CAD build for the part. Positions are in the model's coordinates, mm. A direction names the side the tool comes from. Give positions to 0.01 mm unless a question says otherwise; leave off trailing zeros. Write each loop counter-clockwise with the first axis right and the second up, starting at its lowest first coordinate (ties: lowest second). Pieces come first, ordered by that corner, then holes. Notation, with made-up numbers: (-17, 62.25) -> (39, 62.25) arc R12 cw to (39, 77.25) -> close; hole circle Ø7 at (8, 36.25). An arc over 180 degrees is marked (long way). Answer in a Markdown table with one row per item. Add a question column.
```python
from build123d import *

# Parameters (mm, degrees)
SKETCH_1_W   = 40
SKETCH_1_H   = 10
SKETCH_1_W_2 = 20
SKETCH_1_H_2 = 40
SKETCH_1_H_3 = 2.5


with BuildPart() as part:
    # 草圖1 → 旋轉1 (revolve)
    with BuildSketch(Plane.XY, mode=Mode.PRIVATE) as revolve_1_sk:
        with Locations((-20, 25)):
            Rectangle(SKETCH_1_W, SKETCH_1_H)
        with Locations((10, 20)):
            Rectangle(SKETCH_1_W_2, SKETCH_1_H_2)
        Polygon((20, 25), (20, 0), (40, 0), (40, 20), (40, 25), align=None)
        Polygon((40, 20), (40, 0), (60, 0), (60, 15), (60, 20), align=None)
        Polygon((60, 15), (60, 0), (80, 0), (80, 10), (80, 15), align=None)
        Polygon((80, 10), (80, 0), (100, 0), (100, 5), (100, 10), align=None)
        Polygon((100, 5), (100, 0), (120, 0), (120, 2.5), (120, 5), align=None)
        with Locations((130, 1.25)):
            Rectangle(SKETCH_1_W_2, SKETCH_1_H_3)
    revolve(revolve_1_sk.sketch.rotate(Axis((0, 0, 0), (1, 0, 0)), 90), axis=Axis((0, 0, 0), (1, 0, 0)))


solid = part.part
```
Item 1: Slice it at C-C, the plane x = 114.5. List the corners of the cut face in (y, z), then the cut area to 3 significant figures.
Item 2: Slice it at D-D, the plane y = 34. List the corners of the cut face in (x, z).
Item 3: Probe L1, parallel to Y at x = -16.5, z = 0; L2, parallel to Z at x = -3.5, y = -16; L3, parallel to X at y = -22.5, z = -28.5. List the from-to ranges inside material, lowest first. Write a range as from..to.
Item 4: Which spindle directions (+Z, -Z, +X, -X, +Y, -Y) get a long thin tool onto all of the face, cutting with end or side? Do faces 4 (the face through (140, 0, 0)), 5 (the face through (-19.72, -25.296, 16.128)), 6 (the face through (110, 0, -5)). Say none if no direction does.
Item 5: Mould opens along Y. For faces 1 (the face through (-19.72, -0.88, -19.98)), 2 (the face through (10.14, -1.76, -39.96)), 3 (the face through (20, 17.22, 18.34)) say: released by +Y, released by -Y, zero draft, split by the parting line, or undercut.
Item 6: Slice it at A-A, the plane z = -12. List the corners of the cut face in (x, y), then the cut area to 3 significant figures.
Item 7: Slice it at B-B, the plane x = -13.5. List the corners of the cut face in (y, z).
Item 8: Drop flat-ended pins along their axis: pin 1 Ø3 at (x, y) = (-21, 3.5) entering from -Z; pin 2 Ø8 at (x, y) = (-6, 20.5) entering from -Z; pin 3 Ø6 at (x, y) = (14.5, -4.5) entering from -Z. Give the stop position or say it passes through.
Answer key:
| question | item | result |
|---|---|---|
| 1 | outline | circle Ø10 at (0, 0) |
| 1 | area | 78.5 mm² |
| 2 | outline | (0, -21.07) -> (20, -21.07) -> (20, 21.07) -> (0, 21.07) -> close |
| 3 | L1 | y = -30..-20, 20..30 |
| 3 | L2 | z = -25.38..-12, 12..25.38 |
| 3 | L3 | x = 0..20 |
| 4 | face 4 | +Z, -Z, +X, +Y, -Y |
| 4 | face 5 | -X |
| 4 | face 6 | +X |
| 5 | face 1 | undercut |
| 5 | face 2 | split by the parting line |
| 5 | face 3 | zero draft |
| 6 | outline | (-40, -27.5) -> (0, -27.5) -> (0, -38.16) -> (20, -38.16) -> (20, -21.93) -> (40, -21.93) -> (40, -16) -> (60, -16) -> (60, -9) -> (80, -9) -> (80, 9) -> (60, 9) -> (60, 16) -> (40, 16) -> (40, 21.93) -> (20, 21.93) -> (20, 38.16) -> (0, 38.16) -> (0, 27.5) -> (-40, 27.5) -> (-40, 16) -> (0, 16) -> (0, -16) -> (-40, -16) -> close |
| 6 | area | 4,320 mm² |
| 7 | outline | circle Ø60 at (0, 0); hole circle Ø40 at (0, 0) |
| 8 | pin 1 | stops at z = -29.93 |
| 8 | pin 2 | stops at z = -25.05 |
| 8 | pin 3 | stops at z = -39.97 |
